Work out the finished part from the listing and answer in its coordinate system (mm). A direction names the side the tool comes from. Round coordinates to 2 decimals unless told otherwise and drop trailing zeros. Loops run counter-clockwise (first coordinate to the right, second up) from the corner with the lowest first, then second, coordinate; pieces in that order, holes last. Notation, with made-up numbers: (22, 73) -> (65, 73) arc R19 cw to (65, 88) -> close; hole circle Ø1 at (62.5, -17). An arc over 180 degrees is marked (long way). Write item = value, one per line. Start each with the question number.
```python
from build123d import *

# Parameters (mm, degrees)
F0_W      = 7.5
F0_H      = 20
F2_DEPTH  = 9.25
F4_DEPTH  = 40
F7_DEPTH  = 5
F9_W      = 17.5
F9_H      = 15
F10_DEPTH = 20


with BuildPart() as f1:
    # F0 (on Front) → F1 (revolve)
    with BuildSketch(Plane.XZ):
        Polygon((18.4253171254, 42.021107682), (23.7392311672, 27.021107682), (23.7392311672, 67.021107682), align=None)
    revolve(axis=Axis((16.2392311672, 0, 39.521107682), (0, 0, 1)))


with BuildPart() as f1b:
    # F0 (on Front) → F1, piece 2 (revolve)
    with BuildSketch(Plane.XZ):
        Polygon((22.399485205, 72.021107682), (23.7392311672, 67.021107682), (23.7392311672, 72.021107682), align=None)
        Polygon((23.7392311672, 72.021107682), (23.7392311672, 67.021107682), (26.2392311672, 67.021107682), align=None)
    revolve(axis=Axis((16.2392311672, 0, 39.521107682), (0, 0, 1)))

    # F6 (on face) → F7 (cut, through all)
    with BuildSketch(Plane(origin=(0, 0, 67.021107682), x_dir=(1, 0, 0), z_dir=(0, 0, -1))):
        with BuildLine():
            Line((12.4395601288, 9.25), (20.0389022056, 9.25))
            ThreePointArc((20.0389022056, 9.25), (16.2392311672, 10), (12.4395601288, 9.25))
        make_face()
        with BuildLine():
            ThreePointArc((12.4395601288, -9.25), (16.2392311672, -10), (20.0389022056, -9.25))
            Line((20.0389022056, -9.25), (12.4395601288, -9.25))
        make_face()
    extrude(amount=-F7_DEPTH, mode=Mode.SUBTRACT)


with BuildPart() as f2:
    # F0 (on Front) → F2 (new body, symmetric)
    with BuildSketch(Plane.XZ):
        Polygon((6.2392311672, 7.021107682), (8.7392311672, 7.021107682), (8.7392311672, 27.021107682), (8.7392311672, 67.021107682), (6.2392311672, 67.021107682), align=None)
        Polygon((23.7392311672, 27.021107682), (23.7392311672, 7.021107682), (26.2392311672, 7.021107682), (26.2392311672, 67.021107682), (23.7392311672, 67.021107682), align=None)
        with Locations((12.4892311672, 17.021107682)):
            Rectangle(F0_W, F0_H)
        with Locations((19.9892311672, 17.021107682)):
            Rectangle(F0_W, F0_H)
    extrude(amount=F2_DEPTH, both=True)


with BuildPart() as f4:
    # F3 (on face) → F4 (new body, through all)
    with BuildSketch(Plane.XY.offset(27.021107682)):
        with BuildLine():
            Line((23.7392311672, -9.25), (23.7392311672, 0))
            ThreePointArc((23.7392311672, 0), (16.2392311556, -7.5), (8.7392311672, 2.31e-08))
            Line((8.7392311672, 2.31e-08), (8.7392311672, -9.25))
            Line((8.7392311672, -9.25), (23.7392311672, -9.25))
        make_face()
    extrude(amount=F4_DEPTH)


with BuildPart() as f4b:
    # F3 (on face) → F4, piece 2 (new body, through all)
    with BuildSketch(Plane.XY.offset(27.021107682)):
        with BuildLine():
            Line((23.7392311672, 0), (23.7392311672, 9.25))
            Line((23.7392311672, 9.25), (8.7392311672, 9.25))
            Line((8.7392311672, 9.25), (8.7392311672, 2.31e-08))
            ThreePointArc((8.7392311672, 2.31e-08), (16.2392311787, 7.5), (23.7392311672, 0))
        make_face()
    extrude(amount=F4_DEPTH)


with BuildPart() as f4_1:
    add(f4.part)

    # F8: union F1b, F2, F1, F4b
    add(f1b.part)
    add(f2.part)
    add(f1.part)
    add(f4b.part)

    # F9 (on face) → F10 (cut)
    with BuildSketch(Plane(origin=(0, 0, 7.021107682), x_dir=(1, 0, 0), z_dir=(0, 0, -1))):
        with Locations((16.2392311672, 0)):
            Rectangle(F9_W, F9_H)
    extrude(amount=-F10_DEPTH, mode=Mode.SUBTRACT)


solid = f4_1.part
```
Item 1: Section A-A (z = 11) is taken. Determine the outline of the cut face in (x, y), then the cut area to 4 significant figures.
Item 2: The mould has two halves that part along Y. Classify faces 1 (the flat face through (6.239, 0, 37)), 2 (the flat face through (24.989, 0, 17)), 3 (the conical face through (23.509, 2.289, 71.778)): pulls with the +Y half, pulls with the -Y half, needs draft (parallel to the pull), parting line crosses it, or undercut.
Item 3: Find the intervals of material crossed by line 1 along X through (y, z) = (4, 26); line 2 along Z through (x, y) = (7, -5.5); line 3 along Y through (x, z) = (21.75, 17), in increasing order. Write a range as [from, to].
Item 4: Section C-C (z = 46) is taken. Determine the outline of the cut face in (x, y), then the cut area to 3 significant figures.
Item 5: Section B-B (z = 30.5) is taken. Determine the outline of the cut face in (x, y), then the cut area to 3 significant figures.
Item 6: A tool of negligible diameter and unlimited length cuts with its end or side. For faces 4 (the flat face through (25, 7, 67.021)), 5 (the flat face through (8, 7, 67.021)), 6 (the flat face through (8, -7, 67.021)), 7 (the flat face through (8.6, -0.6, 27.021)), from which of +Z, -Z, +X, -X, +Y, -Y can it reach the whole face along a straight path? Write none if from no direction.
Item 7: A flat-ended cylindrical pin translates along its axis: pin 1 (9.5 mm diameter, centred on x = 19, y = -2.5, fed in from -Z). Find the tip coordinate at first contact, or state that the pin passes through.
Worked answers:
q1.outline = (6.24, -9.25) -> (26.24, -9.25) -> (26.24, 9.25) -> (6.24, 9.25) -> close; hole (7.49, -7.5) -> (24.99, -7.5) -> (24.99, 7.5) -> (7.49, 7.5) -> close
q1.area = 107.5 mm2
q2.face_1 = needs draft
q2.face_2 = undercut
q2.face_3 = parting line crosses it
q3.line_1 = [6.24, 7.49], [24.99, 26.24]
q3.line_2 = [7.02, 67.02]
q3.line_3 = [-9.25, -7.5], [7.5, 9.25]
q4.outline = (6.24, -9.25) -> (26.24, -9.25) -> (26.24, 9.25) -> (6.24, 9.25) -> close; hole circle Ø6.06 at (16.24, 0)
q4.area = 341 mm2
q5.outline = (6.24, -9.25) -> (26.24, -9.25) -> (26.24, 9.25) -> (6.24, 9.25) -> close; hole circle Ø12.54 at (16.24, 0)
q5.area = 247 mm2
q6.face_4 = +Z, +X, +Y
q6.face_5 = +Z, -X, +Y
q6.face_6 = +Z, -X, -Y
q6.face_7 = -Z
q7.pin_1 = 27.02
